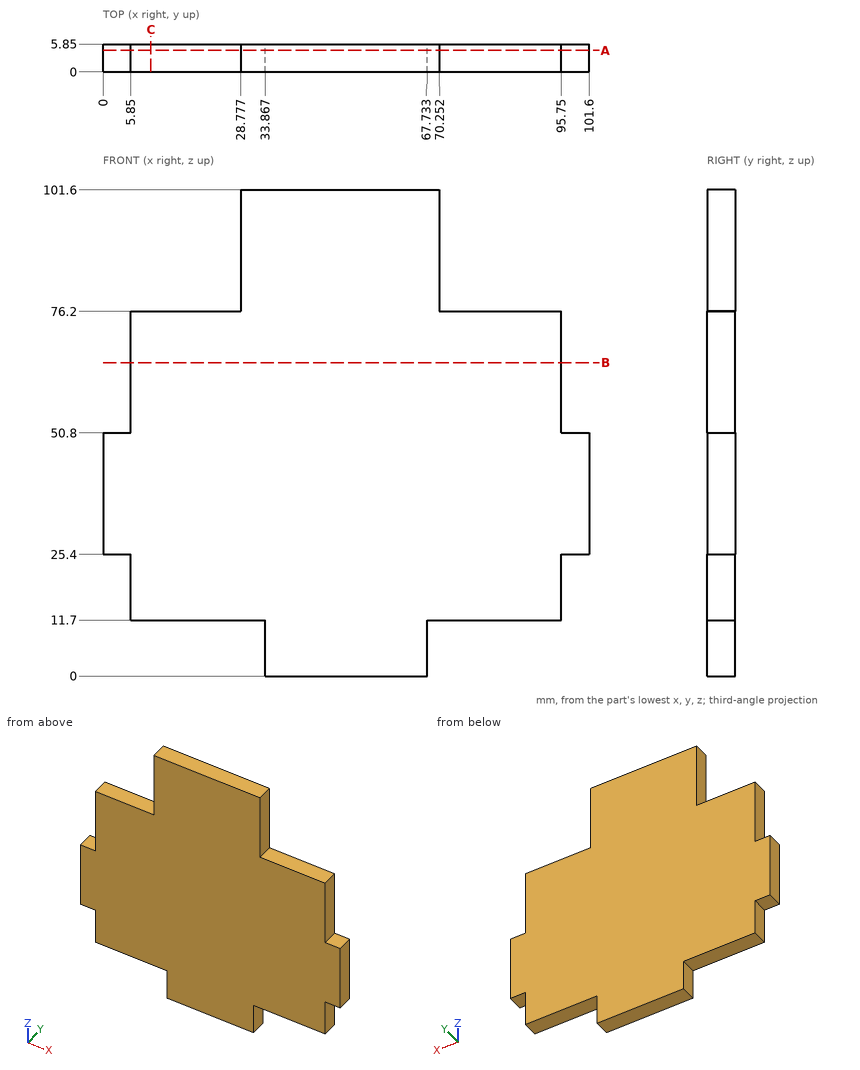
Geometry check sheet. Reference: drawing and pictorial views, mm from the part's lowest x, y, z. Coordinates: 2 decimals unless noted, no trailing zeros. Order: outer loops, then holes, each group sorted by start corner. A loop starts at its lowest first (then second) coordinate and runs counter-clockwise, first axis right, second up. Notation, with made-up numbers: M 30.5,-37 L 61.5,-37 A16 cw 61.5,-19 Z; hole C 31.25,27.25 d7. An arc over 180 degrees is marked long. Write each question's results on one line, items separated by ' | '. Start each with the question number.
1. Cross-section at A-A on y = 4.5. Record the cut outline in (x, z), and give its area (3 significant figures).
2. Go/stop test with flat-tipped pins: P1, Ø1, axis at y = 3, z = 10.5, coming from the +X side; P2, Ø3, axis at y = 4, z = 8.5, coming from the -X side; P3, Ø3, axis at y = 2.5, z = 65, coming from the -X side. Record where each tip stops, or that it passes through.
3. Cross-section at B-B on z = 65.5. Record the cut outline in (x, y), and give its area (3 significant figures).
4. Material ranges on probe 1 along Z at (x, y) = (15, 1); probe 2 along X at (y, z) = (3.7, 61.5); probe 3 along Z at (x, y) = (68, 2.9), recorded low to high.
5. Cross-section at C-C on x = 10. Record the cut outline in (y, z).
Checks:
1) outline: M 0,25.4 L 5.85,25.4 L 5.85,11.7 L 33.87,11.7 L 33.87,0 L 67.73,0 L 67.73,11.7 L 95.75,11.7 L 95.75,25.4 L 101.6,25.4 L 101.6,50.8 L 95.75,50.8 L 95.75,76.2 L 70.25,76.2 L 70.25,101.6 L 28.78,101.6 L 28.78,76.2 L 5.85,76.2 L 5.85,50.8 L 0,50.8 Z | area: 7,550 mm²
2) P1: stops at x = 67.73 | P2: stops at x = 33.87 | P3: stops at x = 5.85
3) outline: M 5.85,0 L 95.75,0 L 95.75,5.85 L 5.85,5.85 Z | area: 526 mm²
4) probe 1: z = 11.7 to 76.2 | probe 2: x = 5.85 to 95.75 | probe 3: z = 11.7 to 101.6
5) outline: M 0,11.7 L 5.85,11.7 L 5.85,76.2 L 0,76.2 Z
